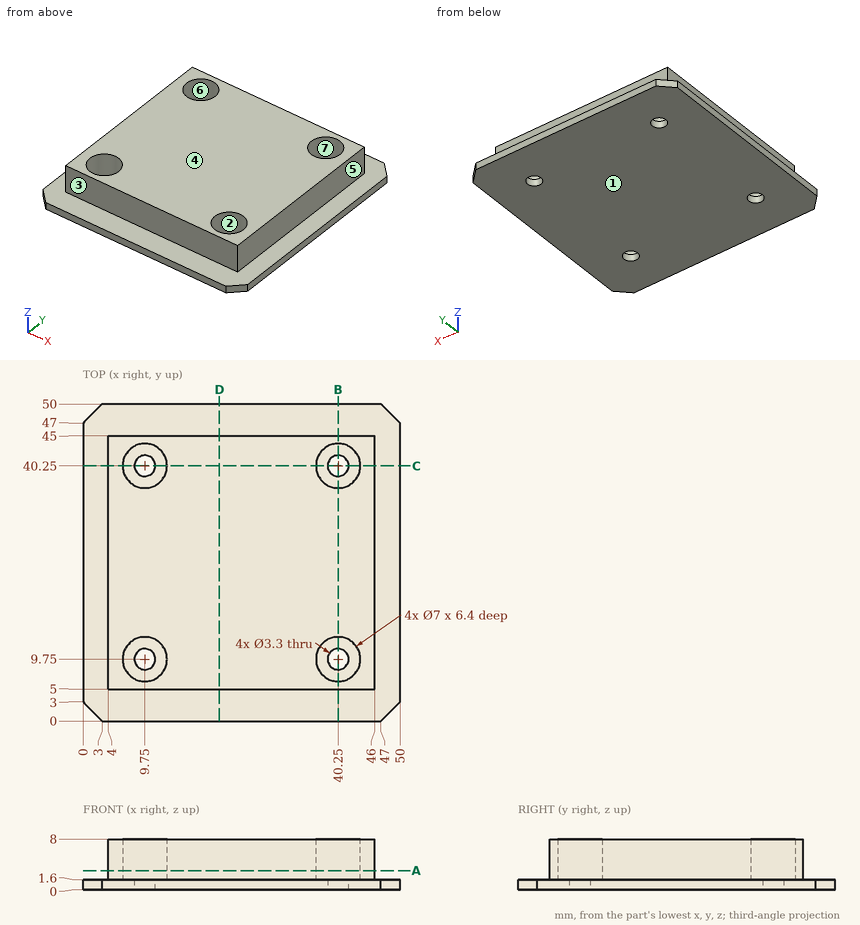
Job drawing, mm, ordinate dimensions from the low corner. One solid piece. A direction names the side the tool comes from. Round coordinates to 2 decimals unless told otherwise and drop trailing zeros. Loops run counter-clockwise (first coordinate to the right, second up) from the corner with the lowest first, then second, coordinate; pieces in that order, holes last. Notation, with made-up numbers: M -28.75,-21 L 27.25,-21 A17 cw 27.25,-8 Z; hole C 17,34 d3. An arc over 180 degrees is marked long. One line per question, with ' | ' between items. Start each with the question number.
Item 1: Cut at D-D, the plane x = 21.5. Write the cut outline in (y, z).
Item 2: Pin check, flat tips, straight feed: pin 1 Ø3 at (y, z) = (25.5, 5) entering from -X; pin 2 Ø1 at (x, y) = (38.5, 41.5) entering from +Z; pin 3 Ø4 at (x, z) = (17.5, 5) entering from +Y; pin 4 Ø3 at (x, y) = (40.25, 9.75) entering from +Z. Stop position of each tip, or through.
Item 3: Cut at B-B, the plane x = 40.25. Write the cut outline in (y, z).
Item 4: Cut at A-A, the plane z = 3. Write the cut outline in (x, y).
Item 5: Two-plate mould, pull along X, no slides. Class the marked faces 4, 5, 6 and 7: pulls with the +X half, pulls with the -X half, needs draft (parallel to the pull), parting line crosses it, or undercut.
Item 6: Wall check: line 1 (Y direction, x = 40.25, z = 1.05); line 2 (X direction, y = 8, z = 2); line 3 (Z direction, x = 34, y = 3.5). Give the ranges that are in metal, low to high.
Item 7: Cut at C-C, the plane y = 40.25. Write the cut outline in (x, z).
Item 8: Which spindle directions (+Z, -Z, +X, -X, +Y, -Y) get a long thin tool onto all of the face, cutting with end or side? Do the marked faces 1, 2 and 3. Say none if no direction does.
Responses:
1) outline: M 0,0 L 50,0 L 50,1.6 L 45,1.6 L 45,8 L 5,8 L 5,1.6 L 0,1.6 Z
2) pin 1: stops at x = 4 | pin 2: stops at z = 1.6 | pin 3: stops at y = 45 | pin 4: passes through
3) outline: M 0,0 L 8.1,0 L 8.1,1.6 L 6.25,1.6 L 6.25,8 L 5,8 L 5,1.6 L 0,1.6 Z; M 11.4,0 L 38.6,0 L 38.6,1.6 L 36.75,1.6 L 36.75,8 L 13.25,8 L 13.25,1.6 L 11.4,1.6 Z; M 41.9,0 L 50,0 L 50,1.6 L 45,1.6 L 45,8 L 43.75,8 L 43.75,1.6 L 41.9,1.6 Z
4) outline: M 4,5 L 46,5 L 46,45 L 4,45 Z; hole C 9.75,9.75 d7; hole C 9.75,40.25 d7; hole C 40.25,9.75 d7; hole C 40.25,40.25 d7
5) face 4: needs draft | face 5: pulls with the +X half | face 6: undercut | face 7: undercut
6) line 1: y = 0 to 8.1, 11.4 to 38.6, 41.9 to 50 | line 2: x = 4 to 6.72, 12.78 to 37.22, 43.28 to 46 | line 3: z = 0 to 1.6
7) outline: M 0,0 L 8.1,0 L 8.1,1.6 L 6.25,1.6 L 6.25,8 L 4,8 L 4,1.6 L 0,1.6 Z; M 11.4,0 L 38.6,0 L 38.6,1.6 L 36.75,1.6 L 36.75,8 L 13.25,8 L 13.25,1.6 L 11.4,1.6 Z; M 41.9,0 L 50,0 L 50,1.6 L 46,1.6 L 46,8 L 43.75,8 L 43.75,1.6 L 41.9,1.6 Z
8) face 1: -Z, +X, -X, +Y, -Y | face 2: +Z | face 3: +Z, +X, -X, -Y
